Model file for the job. Use its own axes, mm. A direction names the side the tool comes from. Round coordinates to 2 decimals unless told otherwise and drop trailing zeros. Order: outer loops, then holes, each group sorted by start corner. A loop starts at its lowest first (then second) coordinate and runs counter-clockwise, first axis right, second up. Notation, with made-up numbers: M -10,-3 L 45,-3 A24 ccw 45,22 Z; hole C 44,75.25 d5. An arc over 180 degrees is marked long. Return JSON: item names as keys, results as strings. Group by question number.
Item 1: Probe line 1 along Y through (x, z) = (16, 0.5); line 2 along Y through (x, z) = (0, 2.4) (1 decimal); line 3 along X through (y, z) = (-2, 0.55). List the from-to ranges inside material, lowest first.
Item 2: Slice it at D-D on y = 10. Write the cut outline in (x, z).
Item 3: Pull direction X, two halves, no side cores. Call faces 3 (the face through (29.43, 0, 2)), 4 (the face through (-20.213, 17.672, 1.607)), 5 (the face through (17, 22.5, 2)), 6 (the face through (-14.944, 0.543, 1.607)): pulls with the +X half, pulls with the -X half, needs draft (parallel to the pull), parting line crosses it, or undercut.
Item 4: Which spindle directions (+Z, -Z, +X, -X, +Y, -Y) get a long thin tool onto all of the face, cutting with end or side? Do faces 1 (the face through (17, -2.5, 2)), 2 (the face through (-11.12, -25.963, 1.563)). Say none if no direction does.
Item 5: Slice it at A-A on y = 0. Write the cut outline in (x, z) (1 decimal).
Item 6: Pin check, flat tips, straight feed: pin 1 Ø8 at (x, y) = (2, 0) entering from +Z; pin 2 Ø1 at (y, z) = (-14, 1) entering from -X (3 decimals). Stop position of each tip, or through.
Item 7: Slice it at B-B on x = 0. Write the cut outline in (y, z) (1 decimal).
Item 8: Slice it at C-C on x = 17. Write the cut outline in (y, z), then the cut area to 3 significant figures.
Autodesk Inventor part; units mm, degrees
ref_plane "YZ Plane" through (0, 0, 0) normal (1, 0, 0) x (0, 1, 0)
ref_plane "XZ Plane" through (0, 0, 0) normal (0, 1, 0) x (-1, 0, 0)
ref_plane "XY Plane" through (0, 0, 0) normal (0, 0, 1) x (1, 0, 0)
sketch "Sketch1" plane through (0, 0, 0) normal (0, 0, 1) x (1, 0, 0)
  line L0 (-29.86, 26.5) -> (29.43, 26.5)
  line L1 (29.43, 26.5) -> (29.43, -26.5)
  line L2 (29.43, -26.5) -> (-29.86, -26.5)
  line L3 (-29.86, -26.5) -> (-29.86, 26.5)
  line L4 (-29.86, 0) -> (29.43, 0) construction
  circle A0 centre (0, 0) radius 5.5
  dimension "d0" = 29.86
  dimension "d1" = 59.29
  dimension "d2" = 53
  dimension "d3" = 11
extrude "Extrusion1" add sketch "Sketch1" along normal blind 3.17
sketch "Sketch2" plane through (0, 0, 3.17) normal (0, 0, 1) x (1, 0, 0)
  circle A0 centre (0, 0) radius 5.5
  line L0 (29.43, -26.5) -> (29.43, 26.5)
  line L1 (0, 0) -> (0, 49.2966)
  circle A1 centre (0, 16.6681) radius 1.8076
  circle A2 centre (-16.6681, 0) radius 1.8076
  circle A3 centre (0, -16.6681) radius 1.8076
  dimension "d8" = 180
extrude "Extrusion2" cut sketch "Sketch2" against normal up to next contours A1 L1 | L1 A1 | A2 | A3
sketch "Sketch3" plane through (0, 0, 3.17) normal (0, 0, 1) x (1, 0, 0)
  circle A0 centre (0, 0) radius 5.5
  circle A1 centre (0, 0) radius 8.025
  dimension "d12" = 16.05
extrude "Extrusion3" cut sketch "Sketch3" against normal blind 2
sketch "Sketch4" plane through (0, 0, 3.17) normal (0, 0, 1) x (1, 0, 0)
  line L0 (29.43, 26.5) -> (-29.86, 26.5)
  line L1 (-29.86, 26.5) -> (-29.86, -26.5)
  line L2 (29.43, -26.5) -> (29.43, 26.5)
  line L3 (14, 0) -> (19.9977, 0) construction
  line L4 (14, -2.5) -> (19.9977, -2.5)
  line L5 (19.9977, 2.5) -> (14, 2.5)
  arc A0 (14, 2.5) -> (14, -2.5) centre (14, 0) ccw
  arc A1 (19.9977, -2.5) -> (19.9977, 2.5) centre (19.9977, 0) ccw
  line L6 (14, 10) -> (19.9977, 10) construction
  line L7 (14, 7.5) -> (19.9977, 7.5)
  line L8 (19.9977, 12.5) -> (14, 12.5)
  arc A2 (14, 12.5) -> (14, 7.5) centre (14, 10) ccw
  arc A3 (19.9977, 7.5) -> (19.9977, 12.5) centre (19.9977, 10) ccw
  line L9 (14, 20) -> (19.9977, 20) construction
  line L10 (14, 17.5) -> (19.9977, 17.5)
  line L11 (19.9977, 22.5) -> (14, 22.5)
  arc A4 (14, 22.5) -> (14, 17.5) centre (14, 20) ccw
  arc A5 (19.9977, 17.5) -> (19.9977, 22.5) centre (19.9977, 20) ccw
  line L12 (14, -10) -> (19.9977, -10) construction
  line L13 (14, -12.5) -> (19.9977, -12.5)
  line L14 (19.9977, -7.5) -> (14, -7.5)
  arc A6 (14, -7.5) -> (14, -12.5) centre (14, -10) ccw
  arc A7 (19.9977, -12.5) -> (19.9977, -7.5) centre (19.9977, -10) ccw
  line L15 (14, 0) -> (19.9977, 0) construction
  line L16 (14, -2.5) -> (19.9977, -2.5)
  line L17 (19.9977, 2.5) -> (14, 2.5)
  arc A8 (14, 2.5) -> (14, -2.5) centre (14, 0) ccw
  arc A9 (19.9977, -2.5) -> (19.9977, 2.5) centre (19.9977, 0) ccw
  line L18 (14, 10) -> (19.9977, 10) construction
  line L19 (14, 7.5) -> (19.9977, 7.5)
  line L20 (19.9977, 12.5) -> (14, 12.5)
  arc A10 (14, 12.5) -> (14, 7.5) centre (14, 10) ccw
  arc A11 (19.9977, 7.5) -> (19.9977, 12.5) centre (19.9977, 10) ccw
  line L21 (14, -20) -> (19.9977, -20) construction
  line L22 (14, -22.5) -> (19.9977, -22.5)
  line L23 (19.9977, -17.5) -> (14, -17.5)
  arc A12 (14, -17.5) -> (14, -22.5) centre (14, -20) ccw
  arc A13 (19.9977, -22.5) -> (19.9977, -17.5) centre (19.9977, -20) ccw
  line L24 (14, -10) -> (19.9977, -10) construction
  line L25 (14, -12.5) -> (19.9977, -12.5)
  line L26 (19.9977, -7.5) -> (14, -7.5)
  arc A14 (14, -7.5) -> (14, -12.5) centre (14, -10) ccw
  arc A15 (19.9977, -12.5) -> (19.9977, -7.5) centre (19.9977, -10) ccw
  line L27 (14, 0) -> (19.9977, 0) construction
  line L28 (14, -2.5) -> (19.9977, -2.5)
  line L29 (19.9977, 2.5) -> (14, 2.5)
  arc A16 (14, 2.5) -> (14, -2.5) centre (14, 0) ccw
  arc A17 (19.9977, -2.5) -> (19.9977, 2.5) centre (19.9977, 0) ccw
  point P0 (16.9988, 0)
  point P1 (16.9988, 10)
  point P2 (16.9988, 20)
  point P3 (16.9988, -10)
  point P4 (16.9988, 0)
  point P5 (16.9988, 10)
  point P6 (16.9988, -20)
  point P7 (16.9988, -10)
  point P8 (16.9988, 0)
  dimension "d15" = 5
  dimension "d16" = 43.86
  dimension "d19" = 10
  dimension "d22" = 10
extrude "Extrusion4" cut sketch "Sketch4" against normal up to next
sketch "Sketch5" plane through (0, 0, 3.17) normal (0, 0, 1) x (1, 0, 0)
  line L0 (29.43, 26.5) -> (-29.86, 26.5)
  line L1 (-29.86, 26.5) -> (-29.86, -26.5)
  line L2 (-29.86, -26.5) -> (29.43, -26.5)
  line L3 (-29.86, 8.025) -> (-11.385, 26.5)
  line L4 (-29.86, 8.025) -> (-3.7324, 8.025) construction
  line L5 (-29.86, -8.025) -> (-11.385, -26.5)
  dimension "d27" = 45
extrude "Extrusion5" cut sketch "Sketch5" against normal up to next
fillet "Fillet1" radius 7.25 2 edges at (-11.385, -26.5, 1.585) (-11.385, 26.5, 1.585)
fillet "Fillet2" radius 10.68 2 edges at (-29.86, -8.025, 1.585) (-29.86, 8.025, 1.585)
fillet "Fillet3" radius 5 2 edges at (29.43, 26.5, 1.585) (29.43, -26.5, 1.585)
properties part number "VSLOT Threaded Rod Plate"
Output values:
{
 "1": {"line 1": "-26.5 to -22.5, -17.5 to -12.5, -7.5 to -2.5, 2.5 to 7.5, 12.5 to 17.5, 22.5 to 26.5", "line 2": "-26.5 to -18.5, -14.9 to -8, 8 to 14.9, 18.5 to 26.5", "line 3": "-29.86 to -5.12, 5.12 to 12.5, 21.5 to 29.43"},
 "2": {"outline": "M -27.73,0 L 11.5,0 L 11.5,3.17 L -27.73,3.17 Z; M 22.5,0 L 29.43,0 L 29.43,3.17 L 22.5,3.17 Z"},
 "3": {"face 3": "pulls with the +X half", "face 4": "pulls with the -X half", "face 5": "undercut", "face 6": "undercut"},
 "4": {"face 1": "+Z, -Z", "face 2": "+Z, -Z, -X, -Y"},
 "5": {"outline": "M -29.9,0 L -18.5,0 L -18.5,3.2 L -29.9,3.2 Z; M -14.9,0 L -5.5,0 L -5.5,1.2 L -8,1.2 L -8,3.2 L -14.9,3.2 Z; M 5.5,0 L 11.5,0 L 11.5,3.2 L 8,3.2 L 8,1.2 L 5.5,1.2 Z; M 22.5,0 L 29.4,0 L 29.4,3.2 L 22.5,3.2 Z"},
 "6": {"pin 1": "z = 1.17", "pin 2": "x = -24.385"},
 "7": {"outline": "M -26.5,0 L -18.5,0 L -18.5,3.2 L -26.5,3.2 Z; M -14.9,0 L -5.5,0 L -5.5,1.2 L -8,1.2 L -8,3.2 L -14.9,3.2 Z; M 5.5,0 L 14.9,0 L 14.9,3.2 L 8,3.2 L 8,1.2 L 5.5,1.2 Z; M 18.5,0 L 26.5,0 L 26.5,3.2 L 18.5,3.2 Z"},
 "8": {"outline": "M -26.5,0 L -22.5,0 L -22.5,3.17 L -26.5,3.17 Z; M -17.5,0 L -12.5,0 L -12.5,3.17 L -17.5,3.17 Z; M -7.5,0 L -2.5,0 L -2.5,3.17 L -7.5,3.17 Z; M 2.5,0 L 7.5,0 L 7.5,3.17 L 2.5,3.17 Z; M 12.5,0 L 17.5,0 L 17.5,3.17 L 12.5,3.17 Z; M 22.5,0 L 26.5,0 L 26.5,3.17 L 22.5,3.17 Z", "area": "88.8 mm²"}
}
